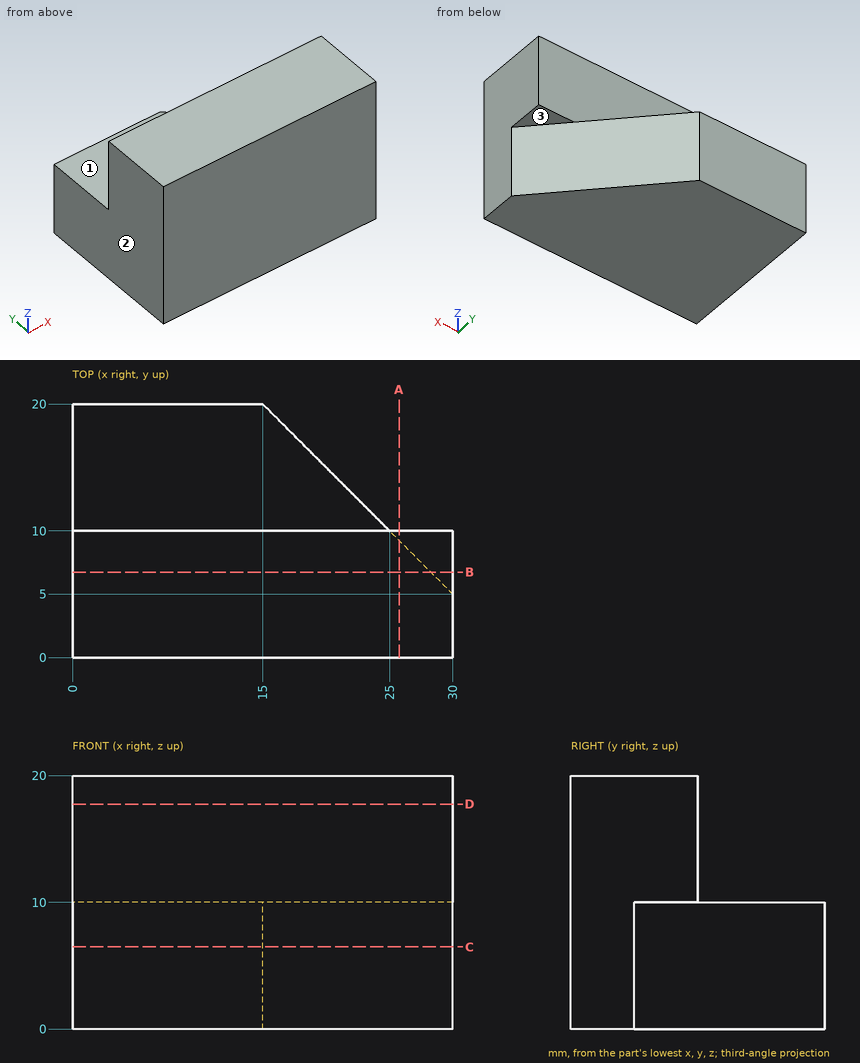
Can you work these out from the drawing? Everything is in mm from the part's minimum corner. A direction names the side the tool comes from. Round coordinates to 2 decimals unless told otherwise and drop trailing zeros. Order: outer loops, then holes, each group sorted by start corner. A loop starts at its lowest first (then second) coordinate and runs counter-clockwise, first axis right, second up. Notation, with made-up numbers: (59, 86) - (71, 86) arc R23 cw to (71, 114) - close; hole circle Ø8 at (68, 36.25). An arc over 180 degrees is marked (long way). Answer in a Markdown table with one row per item.
(1) Suppose I cut it at A-A, the plane x = 25.75. Please give me the cut outline in (y, z), plus the area to 4 significant figures.
From the geometry:
| item | result |
|---|---|
| outline | (0, 0) - (9.25, 0) - (9.25, 10) - (10, 10) - (10, 20) - (0, 20) - close |
| area | 192.5 mm2 |
(2) Which directions (+Z, -Z, +X, -X, +Y, -Y) give clear straight access to the entire face, cutting with the end or side of a thin tool? Please do the marked faces 1, 2 and 3.
From the geometry:
| item | result |
|---|---|
| face 1 | +Z, +X, -X, +Y |
| face 2 | +Z, -Z, -X, +Y, -Y |
| face 3 | -Z, +X, +Y |
(3) Suppose I cut it at B-B, the plane y = 6.75. Please give me the cut outline in (x, z).
From the geometry:
| item | result |
|---|---|
| outline | (0, 0) - (28.25, 0) - (28.25, 10) - (30, 10) - (30, 20) - (0, 20) - close |
(4) Suppose I cut it at D-D, the plane z = 17.75. Please give me the cut outline in (x, y).
From the geometry:
| item | result |
|---|---|
| outline | (0, 0) - (30, 0) - (30, 10) - (0, 10) - close |
(5) Suppose I cut it at C-C, the plane z = 6.5. Please give me the cut outline in (x, y), plus the area to 4 significant figures.
From the geometry:
| item | result |
|---|---|
| outline | (0, 0) - (30, 0) - (30, 5) - (15, 20) - (0, 20) - close |
| area | 487.5 mm2 |
(6) For P1, Ø3, axis at x = 10, y = 14, coming from the +Z side; P2, Ø3, axis at x = 15.5, z = 12.5, coming from the +Y side, each with a flat end and sliding along its axis, tell me the tip position at first contact or that it passes through.
From the geometry:
| item | result |
|---|---|
| P1 | stops at z = 10 |
| P2 | stops at y = 10 |
(7) Please list where these lines run through material, in increasing order: L1, parallel to Z at x = 9.25, y = 11; L2, parallel to X at y = 15, z = 8. Write a range as from..to.
From the geometry:
| item | result |
|---|---|
| L1 | z = 0..10 |
| L2 | x = 0..20 |
